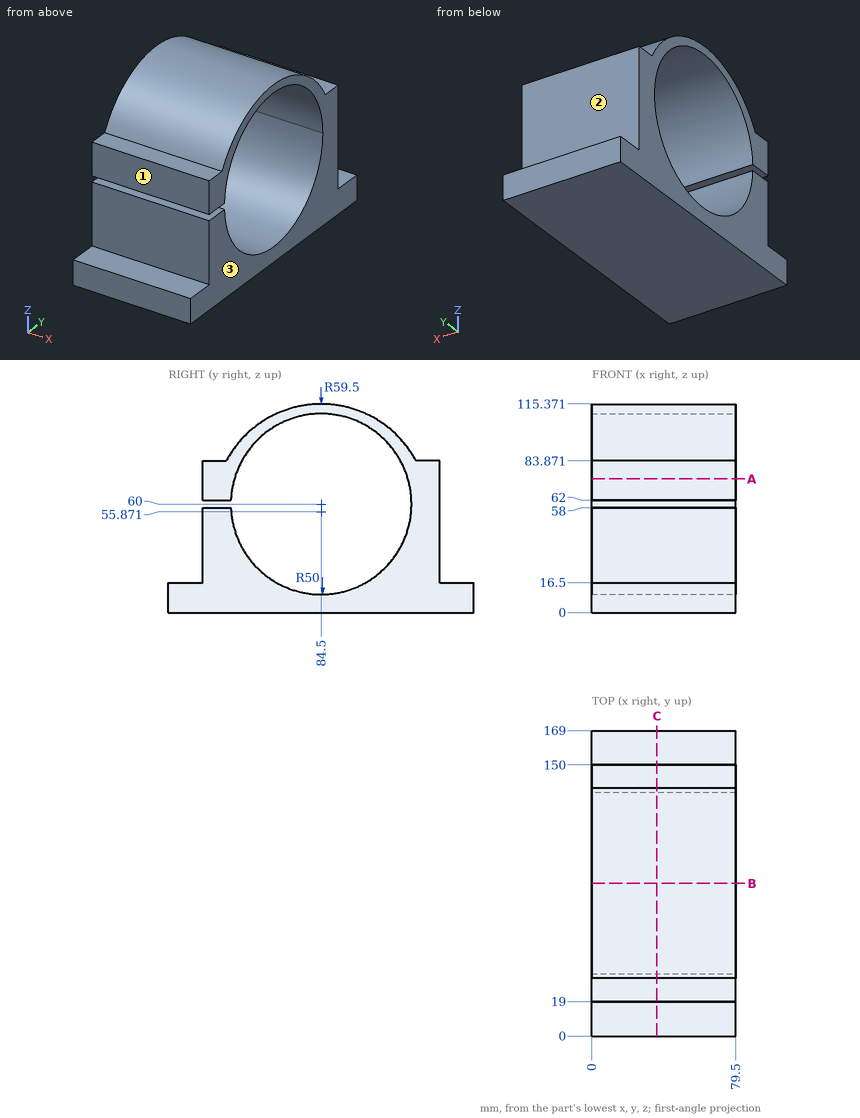
Part print with two shaded views. Sizes in mm from the minimum x, y, z corner. A direction names the side the tool comes from. Coordinates: 2 decimals unless noted, no trailing zeros. Write each loop counter-clockwise with the first axis right and the second up, starting at its lowest first coordinate (ties: lowest second). Pieces come first, ordered by that corner, then holes.
(1) Cut at A-A on z = 74. List the corners of the cut face in (x, y).
(2) Cut at C-C on x = 36. List the corners of the cut face in (y, z).
(3) Drill centre lines: line 1 (Z direction, x = 4, y = 63); line 2 (Z direction, x = 17, y = 106.5) (1 decimal); line 3 (Y direction, x = 44, z = 45). Where is each one in solid material? Low to high.
(4) Pin check, flat tips, straight feed: pin 1 Ø24 at (x, z) = (33, 70.5) entering from -Y; pin 2 Ø5.5 at (x, y) = (36.5, 6) entering from +Z; pin 3 Ø20 at (x, z) = (21, 39) entering from +Y. Stop position of each tip, or through.
(5) 3-axis set-ups, long thin cutter, end or side, ignore diameter. For the marked faces 1, 2 and 3: which of +Z, -Z, +X, -X, +Y, -Y reach the whole face in a straight line?
(6) Cut at B-B on y = 84.5. List the corners of the cut face in (x, z), and give its area (3 significant figures).
Working result:
1. outline: (0, 19) - (79.5, 19) - (79.5, 36.5) - (0, 36.5) - close; (0, 132.5) - (79.5, 132.5) - (79.5, 150) - (0, 150) - close
2. outline: (0, 0) - (169, 0) - (169, 16.5) - (150, 16.5) - (150, 83.87) - (137, 83.87) arc R59.5 ccw to (32, 83.87) - (19, 83.87) - (19, 62) - (34.54, 62) arc R50 cw (long way) to (34.54, 58) - (19, 58) - (19, 16.5) - (0, 16.5) - close
3. line 1: z = 0 to 14.86, 105.14 to 111.35
3. line 2: z = 0 to 15.1, 104.9 to 111.2
3. line 3: y = 19 to 36.8, 132.2 to 150
4. pin 1: stops at y = 19
4. pin 2: stops at z = 16.5
4. pin 3: stops at y = 150
5. face 1: +Z, +X, -X, -Y
5. face 2: +Z, +X, -X, +Y
5. face 3: +Z, -Z, +X, +Y, -Y
6. outline: (0, 0) - (79.5, 0) - (79.5, 10) - (0, 10) - close; (0, 110) - (79.5, 110) - (79.5, 115.37) - (0, 115.37) - close
6. area: 1,220 mm2
